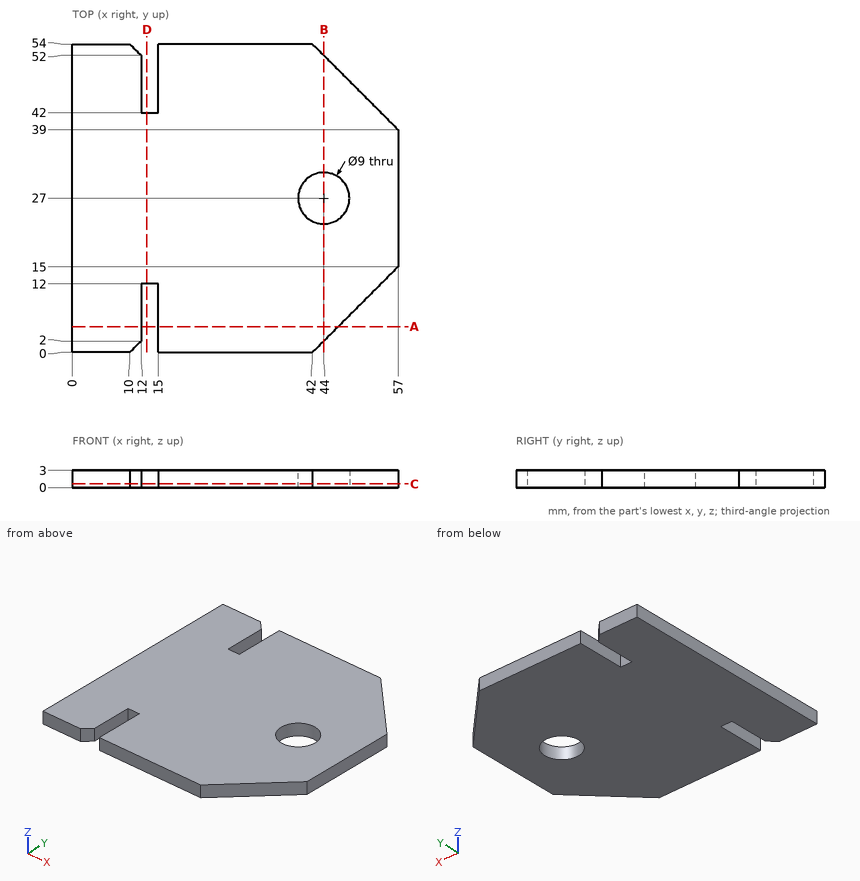
The drawing under review shows one solid part. Ordinate dimensions are in mm from its lowest x, y, z. Give positions to 0.01 mm unless a question says otherwise; leave off trailing zeros. Order: outer loops, then holes, each group sorted by start corner. A loop starts at its lowest first (then second) coordinate and runs counter-clockwise, first axis right, second up. Notation, with made-up numbers: (8.25, -27.75) -> (29.25, -27.75) arc R32 cw to (29.25, 7.25) -> close; hole circle Ø8 at (-23.75, 11.25). An arc over 180 degrees is marked (long way). Write item = value, one per line.
1) Insertion check: pin 1 (1.5 mm diameter, centred on y = 8, z = 1.5, fed in from +X). The pin has a flat end and moves straight along its axis. Give the tip position at first contact, or say it passes through.
Findings:
pin_1 = 50.75
2) We need section B-B, the plane x = 44. Give the boundary of the cut face in (y, z), and give its area (3 significant figures).
Findings:
outline = (2, 0) -> (22.5, 0) -> (22.5, 3) -> (2, 3) -> close; (31.5, 0) -> (52, 0) -> (52, 3) -> (31.5, 3) -> close
area = 123 mm^2
3) We need section D-D, the plane x = 13. Give the boundary of the cut face in (y, z), and give its area (3 significant figures).
Findings:
outline = (12, 0) -> (42, 0) -> (42, 3) -> (12, 3) -> close
area = 90.0 mm^2
4) We need section A-A, the plane y = 4.5. Give the boundary of the cut face in (x, z).
Findings:
outline = (0, 0) -> (12, 0) -> (12, 3) -> (0, 3) -> close; (15, 0) -> (46.5, 0) -> (46.5, 3) -> (15, 3) -> close
5) To check wall thickness, follow L1, parallel to Y at x = 44, z = 1.65; L2, parallel to Y at x = 47, z = 2.65; L3, parallel to X at y = 4.5, z = 2.4. State the ranges of each line that lie inside material, in increasing order. Write a range as from..to.
Findings:
L1 = 2..22.5, 31.5..52
L2 = 5..23.65, 30.35..49
L3 = 0..12, 15..46.5
6) We need section C-C, the plane z = 0.65. Give the boundary of the cut face in (x, y), and give its area (3 significant figures).
Findings:
outline = (0, 0) -> (10, 0) -> (12, 2) -> (12, 12) -> (15, 12) -> (15, 0) -> (42, 0) -> (57, 15) -> (57, 39) -> (42, 54) -> (15, 54) -> (15, 42) -> (12, 42) -> (12, 52) -> (10, 54) -> (0, 54) -> close; hole circle Ø9 at (44, 27)
area = 2,710 mm^2
